Could you check a few things on this model? Use its own coordinates, in mm. Face numbers are marked on the shaded views. Give positions to 0.01 mm unless a question says otherwise; leave off trailing zeros. Use one line per item in the form item = value. Start each with the question number.
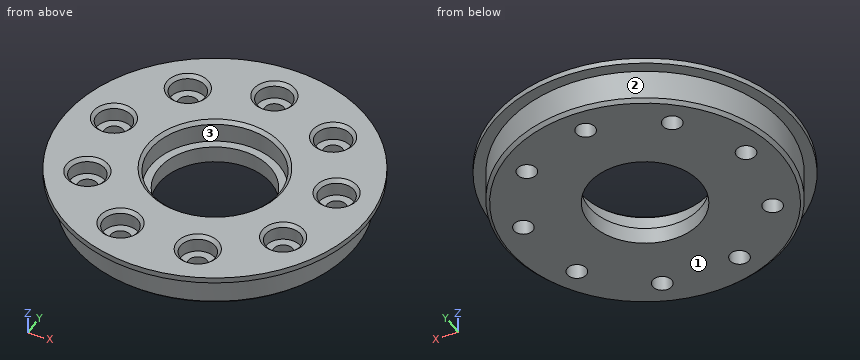
from build123d import *

# Parameters (mm, degrees)
ESQUISSE1_R             = 24.95
BOSS_EXTRU_1_DEPTH      = 6
ESQUISSE2_R             = 26.95
BOSS_EXTRU_2_DEPTH      = 1
ESQUISSE3_R             = 3.1
ENL_V_MAT_EXTRU_1_DEPTH = 3
ESQUISSE4_R             = 1.7
ENL_V_MAT_EXTRU_2_DEPTH = 8
ESQUISSE5_R             = 11.45
ENL_V_MAT_EXTRU_3_DEPTH = 4
ESQUISSE6_R             = 10
ENL_V_MAT_EXTRU_4_DEPTH = 4
CHANFREIN1_SIZE         = 0.6
CHANFREIN2_SIZE         = 0.6


with BuildPart() as part:
    # Esquisse1 → Boss.-Extru.1 (new body)
    with BuildSketch(Plane.XY):
        Circle(ESQUISSE1_R)
    extrude(amount=BOSS_EXTRU_1_DEPTH)

    # Esquisse2 → Boss.-Extru.2 (add)
    with BuildSketch(Plane.XY.offset(6)):
        Circle(ESQUISSE2_R)
    extrude(amount=BOSS_EXTRU_2_DEPTH)

    # Esquisse3 → Enlèv. mat.-Extru.1 (cut)
    with BuildSketch(Plane(origin=(0, 0, 7), x_dir=(-1, 0, 0), z_dir=(0, 0, -1))):
        with Locations((0, 20)):
            Circle(ESQUISSE3_R)
        with Locations((12.855752194, 15.320888862)):
            Circle(ESQUISSE3_R)
        with Locations((19.69615506, 3.472963553)):
            Circle(ESQUISSE3_R)
        with Locations((17.320508076, -10)):
            Circle(ESQUISSE3_R)
        with Locations((6.840402867, -18.793852416)):
            Circle(ESQUISSE3_R)
        with Locations((-6.840402867, -18.793852416)):
            Circle(ESQUISSE3_R)
        with Locations((-17.320508076, -10)):
            Circle(ESQUISSE3_R)
        with Locations((-19.69615506, 3.472963553)):
            Circle(ESQUISSE3_R)
        with Locations((-12.855752194, 15.320888862)):
            Circle(ESQUISSE3_R)
    extrude(amount=ENL_V_MAT_EXTRU_1_DEPTH, mode=Mode.SUBTRACT)

    # Esquisse4 → Enlèv. mat.-Extru.2 (cut, through all)
    with BuildSketch(Plane(origin=(0, 0, 0), x_dir=(-1, 0, 0), z_dir=(0, 0, -1))):
        with Locations((0, 20)):
            Circle(ESQUISSE4_R)
        with Locations((12.855752194, 15.320888862)):
            Circle(ESQUISSE4_R)
        with Locations((19.69615506, 3.472963553)):
            Circle(ESQUISSE4_R)
        with Locations((17.320508076, -10)):
            Circle(ESQUISSE4_R)
        with Locations((6.840402867, -18.793852416)):
            Circle(ESQUISSE4_R)
        with Locations((-6.840402867, -18.793852416)):
            Circle(ESQUISSE4_R)
        with Locations((-17.320508076, -10)):
            Circle(ESQUISSE4_R)
        with Locations((-19.69615506, 3.472963553)):
            Circle(ESQUISSE4_R)
        with Locations((-12.855752194, 15.320888862)):
            Circle(ESQUISSE4_R)
    extrude(amount=-ENL_V_MAT_EXTRU_2_DEPTH, mode=Mode.SUBTRACT)

    # Esquisse5 → Enlèv. mat.-Extru.3 (cut)
    with BuildSketch(Plane.XY.offset(7)):
        Circle(ESQUISSE5_R)
    extrude(amount=-ENL_V_MAT_EXTRU_3_DEPTH, mode=Mode.SUBTRACT)

    # Esquisse6 → Enlèv. mat.-Extru.4 (cut, through all)
    with BuildSketch(Plane.XY.offset(3)):
        Circle(ESQUISSE6_R)
    extrude(amount=-ENL_V_MAT_EXTRU_4_DEPTH, mode=Mode.SUBTRACT)

    # Chanfrein1
    chanfrein1_edges = [part.edges().sort_by_distance(p)[0] for p in [
        (3.1, 20, 7),
        (-9.755752194, 15.320888862, 7),
        (-16.59615506, 3.472963553, 7),
        (-14.220508076, -10, 7),
        (-3.740402867, -18.793852416, 7),
        (9.940402867, -18.793852416, 7),
        (20.420508076, -10, 7),
        (22.79615506, 3.472963553, 7),
        (15.955752194, 15.320888862, 7),
        (-11.45, 0, 7),
    ]]
    chamfer(chanfrein1_edges, length=CHANFREIN1_SIZE)

    # Chanfrein2
    chanfrein2_edges = [part.edges().sort_by_distance(p)[0] for p in [
        (-24.95, 0, 0),
    ]]
    chamfer(chanfrein2_edges, length=CHANFREIN2_SIZE)


solid = part.part
(1) I'm going to push flat-ended pins straight in: pin 1 Ø1 at (x, z) = (-17.5, 5) entering from +Y; pin 2 Ø2 at (y, z) = (7, 6) entering from +X; pin 3 Ø3 at (x, y) = (18.5, -10.5) entering from +Z. Where does each tip first touch, or does it pass through?
(2) Please list where these lines run through material, in increasing order: probe 1 along Y at (x, z) = (-10.5, 6.5); probe 2 along X at (y, z) = (15.5, 1.5); probe 3 along Y at (x, z) = (0.5, 0.5).
(3) We'd pull the mould along Y, two halves only. Please class the marked faces 1, 2 and 3: pulls with the +Y half, pulls with the -Y half, needs draft (parallel to the pull), parting line crosses it, or undercut.
Calculated:
q1.pin_1 = 18.26
q1.pin_2 = 26.27
q1.pin_3 = 4
q2.probe_1 = -24.82 to -4.81, 4.81 to 13.16, 17.49 to 24.82
q2.probe_2 = -19.55 to -14.55, -11.17 to 11.17, 14.55 to 19.55
q2.probe_3 = -24.84 to -9.99, 9.99 to 18.38, 21.62 to 24.84
q3.face_1 = needs draft
q3.face_2 = parting line crosses it
q3.face_3 = undercut
